from build123d import *

# Parameters (mm, degrees)
SKETCH1_W                       = 74
SKETCH1_H                       = 53
BOSS_EXTRUDE1_DEPTH             = 4
SKETCH2_W                       = 3.5
SKETCH2_H                       = 53
BOSS_EXTRUDE2_DEPTH             = 25
CUT_EXTRUDE1_REACH              = 85.781
SKETCH3_W                       = 20
SKETCH3_H                       = 15
SKETCH5_W                       = 20
SKETCH5_H                       = 4
BOSS_EXTRUDE4_DEPTH             = 15
MIRROR4_COPY_1_SKETCH_W         = 20
MIRROR4_COPY_1_SKETCH_H         = 4
MIRROR4_COPY_1_DEPTH            = 15
SKETCH6_W                       = 3.5
SKETCH6_H                       = 15
BOSS_EXTRUDE5_DEPTH             = 25
MIRROR6_COPY_1_SKETCH_W         = 3.5
MIRROR6_COPY_1_SKETCH_H         = 15
MIRROR6_COPY_1_DEPTH            = 25
SKETCH7_W                       = 4.5
SKETCH7_H                       = 12
BOSS_EXTRUDE6_DEPTH             = 7
MIRROR8_COPY_1_SKETCH_W         = 4.5
MIRROR8_COPY_1_SKETCH_H         = 12
MIRROR8_COPY_1_DEPTH            = 7
SKETCH8_W                       = 13
SKETCH8_H                       = 3.5
BOSS_EXTRUDE7_DEPTH             = 16
MIRROR10_COPY_1_SKETCH_W        = 13
MIRROR10_COPY_1_SKETCH_H        = 3.5
MIRROR10_COPY_1_DEPTH           = 16
CUT_EXTRUDE2_REACH              = 105.263
SKETCH9_W                       = 57
SKETCH9_H                       = 15
F_4_0MM_CLEARANCE_DOWEL_HOLE1_D = 4
FILLET1_R                       = 6.5
FILLET2_R                       = 1
FILLET3_R                       = 1


with BuildPart() as part:
    # Sketch1 → Boss-Extrude1 (new body)
    with BuildSketch(Plane(origin=(0, 0, 0), x_dir=(1, 0, 0), z_dir=(0, 1, 0))):
        Rectangle(SKETCH1_W, SKETCH1_H)
    extrude(amount=BOSS_EXTRUDE1_DEPTH)

    # Sketch2 → Boss-Extrude2 (add)
    with BuildSketch(Plane(origin=(0, 4, 0), x_dir=(1, 0, 0), z_dir=(0, 1, 0))):
        with Locations((-35.25, 0)):
            Rectangle(SKETCH2_W, SKETCH2_H)
    boss_extrude2 = extrude(amount=BOSS_EXTRUDE2_DEPTH)

    # Mirror1: Boss-Extrude2 across plane
    add(boss_extrude2.mirror(Plane(origin=(0, 0, 0), x_dir=(0, 0, 1), z_dir=(1, 0, 0))))

    # Sketch3 → Cut-Extrude1 (cut, up to next)
    with BuildSketch(Plane.ZY.offset(37), mode=Mode.PRIVATE) as cut_extrude1_sk1:
        with Locations((0, 21.5)):
            Rectangle(SKETCH3_W, SKETCH3_H)
    cut_extrude1_tool1 = extrude(cut_extrude1_sk1.sketch, amount=-CUT_EXTRUDE1_REACH, mode=Mode.PRIVATE) & part.part
    add(cut_extrude1_tool1.solids().sort_by_distance((-37, 21.5, 0))[0], mode=Mode.SUBTRACT)

    # Sketch5 → Boss-Extrude4 (add)
    with BuildSketch(Plane(origin=(0, 0, -26.5), x_dir=(-1, 0, 0), z_dir=(0, 0, -1))):
        with Locations((27, 2)):
            Rectangle(SKETCH5_W, SKETCH5_H)
    boss_extrude4 = extrude(amount=BOSS_EXTRUDE4_DEPTH)

    # Mirror3: Boss-Extrude4 across plane
    add(boss_extrude4.mirror(Plane.XY))

    # Mirror4: Boss-Extrude4 across plane
    add(boss_extrude4.mirror(Plane(origin=(0, 0, 0), x_dir=(0, 0, 1), z_dir=(1, 0, 0))))

    # Mirror4 copy 1 sketch → Mirror4 copy 1 (add)
    with BuildSketch(Plane.XY.offset(26.5)):
        with Locations((27, 2)):
            Rectangle(MIRROR4_COPY_1_SKETCH_W, MIRROR4_COPY_1_SKETCH_H)
    extrude(amount=MIRROR4_COPY_1_DEPTH)

    # Sketch6 → Boss-Extrude5 (add)
    with BuildSketch(Plane(origin=(0, 4, 0), x_dir=(1, 0, 0), z_dir=(0, 1, 0))):
        with Locations((-35.25, 34)):
            Rectangle(SKETCH6_W, SKETCH6_H)
    boss_extrude5 = extrude(amount=BOSS_EXTRUDE5_DEPTH)

    # Mirror5: Boss-Extrude5 across plane
    add(boss_extrude5.mirror(Plane.XY))

    # Mirror6: Boss-Extrude5 across plane
    add(boss_extrude5.mirror(Plane(origin=(0, 0, 0), x_dir=(0, 0, 1), z_dir=(1, 0, 0))))

    # Mirror6 copy 1 sketch → Mirror6 copy 1 (add)
    with BuildSketch(Plane(origin=(0, 4, 0), x_dir=(-1, 0, 0), z_dir=(0, 1, 0))):
        with Locations((-35.25, 34)):
            Rectangle(MIRROR6_COPY_1_SKETCH_W, MIRROR6_COPY_1_SKETCH_H)
    extrude(amount=MIRROR6_COPY_1_DEPTH)

    # Sketch7 → Boss-Extrude6 (add)
    with BuildSketch(Plane(origin=(0, 4, 0), x_dir=(1, 0, 0), z_dir=(0, 1, 0))):
        with Locations((-23.75, 35.5)):
            Rectangle(SKETCH7_W, SKETCH7_H)
    boss_extrude6 = extrude(amount=BOSS_EXTRUDE6_DEPTH)

    # Mirror7: Boss-Extrude6 across plane
    add(boss_extrude6.mirror(Plane.XY))

    # Mirror8: Boss-Extrude6 across plane
    add(boss_extrude6.mirror(Plane(origin=(0, 0, 0), x_dir=(0, 0, 1), z_dir=(1, 0, 0))))

    # Mirror8 copy 1 sketch → Mirror8 copy 1 (add)
    with BuildSketch(Plane(origin=(0, 4, 0), x_dir=(-1, 0, 0), z_dir=(0, 1, 0))):
        with Locations((-23.75, 35.5)):
            Rectangle(MIRROR8_COPY_1_SKETCH_W, MIRROR8_COPY_1_SKETCH_H)
    extrude(amount=MIRROR8_COPY_1_DEPTH)

    # Sketch8 → Boss-Extrude7 (add)
    with BuildSketch(Plane.ZY.offset(37)):
        with Locations((-35, 27.25)):
            Rectangle(SKETCH8_W, SKETCH8_H)
    boss_extrude7 = extrude(amount=BOSS_EXTRUDE7_DEPTH)

    # Mirror9: Boss-Extrude7 across plane
    add(boss_extrude7.mirror(Plane.XY))

    # Mirror10: Boss-Extrude7 across plane
    add(boss_extrude7.mirror(Plane(origin=(0, 0, 0), x_dir=(0, 0, 1), z_dir=(1, 0, 0))))

    # Mirror10 copy 1 sketch → Mirror10 copy 1 (add)
    with BuildSketch(Plane(origin=(37, 0, 0), x_dir=(0, 0, -1), z_dir=(1, 0, 0))):
        with Locations((-35, 27.25)):
            Rectangle(MIRROR10_COPY_1_SKETCH_W, MIRROR10_COPY_1_SKETCH_H)
    extrude(amount=MIRROR10_COPY_1_DEPTH)

    # Sketch9 → Cut-Extrude2 (cut, up to next)
    with BuildSketch(Plane(origin=(37, 0, 0), x_dir=(0, 0, -1), z_dir=(1, 0, 0)), mode=Mode.PRIVATE) as cut_extrude2_sk1:
        with Locations((0, 21.5)):
            Rectangle(SKETCH9_W, SKETCH9_H)
    cut_extrude2_tool1 = extrude(cut_extrude2_sk1.sketch, amount=-CUT_EXTRUDE2_REACH, mode=Mode.PRIVATE) & part.part
    add(cut_extrude2_tool1.solids().sort_by_distance((37, 21.5, 0))[0], mode=Mode.SUBTRACT)

    # Ø4.0mm Clearance Dowel Hole1 (through all)
    with Locations(Plane(origin=(0, 25.5, 0), x_dir=(-1, 0, 0), z_dir=(0, -1, 0))):
        with Locations((-45, 35), (-45, -35), (45, 35), (45, -35)):
            Hole(F_4_0MM_CLEARANCE_DOWEL_HOLE1_D / 2)

    # Fillet1
    # the kernel refuses this fillet: 6.5 mm, written as the material it takes off along each edge
    with BuildSketch(Plane(origin=(53, 45.25, -28.5), x_dir=(0, 0, -1), z_dir=(0, -1, 0)), Plane(origin=(53, 45.25, 28.5), x_dir=(-1, 0, 0), z_dir=(0, -1, 0)), Plane(origin=(53, 9.25, 41.5), x_dir=(-1, 0, 0), z_dir=(0, 1, 0)), Plane(origin=(-53, 9.25, -41.5), x_dir=(1, 0, 0), z_dir=(0, 1, 0)), Plane(origin=(-53, 45.25, -28.5), x_dir=(1, 0, 0), z_dir=(0, -1, 0))) as fillet1_piece_1:
        with BuildLine():
            CenterArc((FILLET1_R, -FILLET1_R), FILLET1_R, 90, 90)
            Line((0, -FILLET1_R), (0, 0))
            Line((0, 0), (FILLET1_R, 0))
        make_face()
    extrude(amount=36, mode=Mode.SUBTRACT)
    with BuildSketch(Plane(origin=(53, 9.25, -41.5), x_dir=(-1, 0, 0), z_dir=(0, 1, 0)), Plane(origin=(-53, 45.25, 28.5), x_dir=(1, 0, 0), z_dir=(0, -1, 0)), Plane(origin=(-53, 9.25, 41.5), x_dir=(1, 0, 0), z_dir=(0, 1, 0))) as fillet1_piece_2:
        with BuildLine():
            CenterArc((FILLET1_R, FILLET1_R), FILLET1_R, 180, 90)
            Line((0, FILLET1_R), (0, 0))
            Line((0, 0), (FILLET1_R, 0))
        make_face()
    extrude(amount=36, mode=Mode.SUBTRACT)

    # Fillet2
    fillet2_edges = [part.edges().sort_by_distance(p)[0] for p in [
        (-33.5, 4, 0),
        (-37, 25.5, -35),
        (-37, 25.5, 35),
        (37, 25.5, 35),
        (37, 25.5, -35),
        (35.25, 14, 28.5),
        (35.25, 14, -28.5),
        (33.5, 4, 0),
        (-35.25, 14, -10),
        (-35.25, 14, 10),
        (-17, 2, -26.5),
        (-17, 2, 26.5),
        (17, 2, 26.5),
        (17, 2, -26.5),
    ]]
    fillet(fillet2_edges, radius=FILLET2_R)

    # Fillet3
    fillet3_edges = [part.edges().sort_by_distance(p)[0] for p in [
        (0, 0, -26.5),
        (0, 0, 26.5),
        (16.707106781, 0, -26.792893219),
        (-16.707106781, 0, -26.792893219),
        (-16.707106781, 0, 26.792893219),
        (16.707106781, 0, 26.792893219),
        (-37, 0, 0),
        (37, 0, 0),
        (-17, 0, -34.5),
        (-17, 0, 34.5),
        (17, 0, 34.5),
        (17, 0, -34.5),
    ]]
    fillet(fillet3_edges, radius=FILLET3_R)


solid = part.part
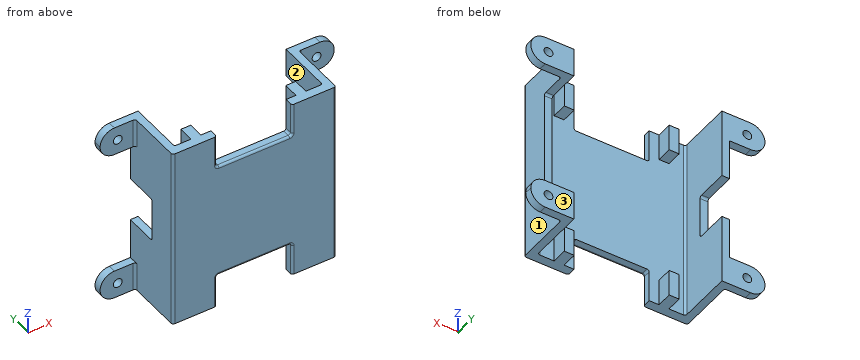
Read the model definition and answer for the solid it produces. Units are mm, in the model's axes. Face numbers are marked on the shaded views. A direction names the side the tool comes from. Give positions to 0.01 mm unless a question says otherwise; leave off trailing zeros. Write each loop counter-clockwise with the first axis right and the second up, starting at its lowest first coordinate (ties: lowest second). Pieces come first, ordered by that corner, then holes. Notation, with made-up numbers: (21, -12.5) - (67, -12.5) arc R20 cw to (67, 23.5) - close; hole circle Ø5 at (87, 57.25). An arc over 180 degrees is marked (long way). Answer in a Markdown table with one row per item. Add a question column.
Item 1: Flat-ended cylindrical pins translate along their axes: P1, Ø3.5, axis at x = -23, z = 36.5, coming from the +Y side; P2, Ø12, axis at x = -24, z = 12, coming from the +Y side; P3, Ø10, axis at y = 18.5, z = -2, coming from the -X side. Find the tip coordinate at first contact, or state that the pin passes through.
Item 2: A tool of negligible diameter and unlimited length cuts with its end or side. For the marked faces 1, 2 and 3, from which of +Z, -Z, +X, -X, +Y, -Y can it reach the whole face along a straight path? Write none if from no direction.
Item 3: Find the intervals of material crossed by L1, parallel to X at y = 28.05, z = -35; L2, parallel to Z at x = -45, y = 27.6; L3, parallel to X at y = 13, z = -19, in increasing order.
Item 4: Section A-A, the plane x = -45 is taken. Write down the section's boundary in (y, z).
Item 5: Section C-C, the plane x = 30.5 is taken. Write down the section's boundary in (y, z).
Item 6: Section B-B, the plane y = 19.75 is taken. Write down the section's boundary in (x, z).
Recorded:
| question | item | result |
|---|---|---|
| 1 | P1 | stops at y = 11 |
| 1 | P2 | stops at y = 4 |
| 1 | P3 | stops at x = -37 |
| 2 | face 1 | +Z, -Z, +X, -Y |
| 2 | face 2 | +Z, -Z, +Y |
| 2 | face 3 | +Z, -Z, +X, -X, +Y |
| 3 | L1 | x = -53 to -47, -43 to -33.5, 33.5 to 43, 47 to 53 |
| 3 | L2 | z = -41.5 to -37, -33 to -28.5, 28.5 to 33, 37 to 41.5 |
| 3 | L3 | x = -37 to -33.5, 33.5 to 37 |
| 4 | outline | (25.5, -41.5) - (29, -41.5) - (29, -37) - (25.5, -37) - close; (25.5, -33) - (29, -33) - (29, -28.5) - (25.5, -28.5) - close; (25.5, 28.5) - (29, 28.5) - (29, 33) - (25.5, 33) - close; (25.5, 37) - (29, 37) - (29, 41.5) - (25.5, 41.5) - close |
| 5 | outline | (0, -41.5) - (4, -41.5) - (4, 41.5) - (0, 41.5) - close |
| 6 | outline | (-37, -41.5) - (-33.5, -41.5) - (-33.5, -10) - (-37, -10) - close; (-37, 10) - (-33.5, 10) - (-33.5, 41.5) - (-37, 41.5) - close; (33.5, -41.5) - (37, -41.5) - (37, -28.5) - (33.5, -28.5) - close; (33.5, 28.5) - (37, 28.5) - (37, 41.5) - (33.5, 41.5) - close |
